```python
from build123d import *

# Parameters (mm, degrees)
SKETCH_1_R           = 4.1
EXTRUDE_1_DEPTH      = 18
EXTRUDE_1_DEPTH_BACK = 18
SKETCH_3_W           = 40
SKETCH_3_H           = 60
EXTRUDE_2_DEPTH      = 4
CUT_EXTRUDE_START    = 50
SKETCH_4_W           = 18
SKETCH_4_H           = 20
CUT_EXTRUDE_1_DEPTH  = 29
SKETCH_5_R           = 6
CUT_EXTRUDE_2_DEPTH  = 55
EXTRUDE_START        = 18
EXTRUDE_3_DEPTH      = 4
EXTRUDE_START_2      = -18
EXTRUDE_4_DEPTH      = 4
SKETCH_7_R           = 2.5
CUT_EXTRUDE_4_DEPTH  = 5
FILLET_1_R           = 2


with BuildPart() as part:
    # Эскиз1 → Бобышка-Вытянуть1 (new body, two sides)
    with BuildSketch(Plane.XY) as extrude_1_sk:
        with BuildLine():
            Line((-9, 0), (-9, -73))
            Line((-9, -73), (9, -73))
            Line((9, -73), (9, 0))
            ThreePointArc((9, 0), (0, 9), (-9, 0))
        make_face()
        Circle(SKETCH_1_R, mode=Mode.SUBTRACT)
    extrude(amount=EXTRUDE_1_DEPTH)
    extrude(extrude_1_sk.sketch, amount=-EXTRUDE_1_DEPTH_BACK)

    # Эскиз3 → Бобышка-Вытянуть2 (add)
    with BuildSketch(Plane.XZ.offset(73)):
        Rectangle(SKETCH_3_W, SKETCH_3_H)
    extrude(amount=-EXTRUDE_2_DEPTH)

    # Эскиз4 → Вырез-Вытянуть1 (cut, through all)
    with BuildSketch(Plane(origin=(0, -69, 0), x_dir=(1, 0, 0), z_dir=(0, 1, 0)).offset(CUT_EXTRUDE_START)):
        Rectangle(SKETCH_4_W, SKETCH_4_H)
    extrude(amount=CUT_EXTRUDE_1_DEPTH, mode=Mode.SUBTRACT)

    # Эскиз5 → Вырез-Вытянуть2 (cut, through all)
    with BuildSketch(Plane(origin=(0, -19, 0), x_dir=(1, 0, 0), z_dir=(0, 1, 0))):
        Circle(SKETCH_5_R)
    extrude(amount=-CUT_EXTRUDE_2_DEPTH, mode=Mode.SUBTRACT)

    # Эскиз6 → Бобышка-Вытянуть3 (add)
    with BuildSketch(Plane.XY.offset(EXTRUDE_START)):
        Polygon((-20, -69), (-9, -34.5), (-9, -69), align=None)
        Polygon((9, -34.5), (20, -69), (9, -69), align=None)
    extrude(amount=-EXTRUDE_3_DEPTH)

    # Эскиз6<3> → Бобышка-Вытянуть4 (add)
    with BuildSketch(Plane.XY.offset(EXTRUDE_START_2)):
        Polygon((-20, -69), (-9, -34.5), (-9, -69), align=None)
        Polygon((9, -34.5), (20, -69), (9, -69), align=None)
    extrude(amount=EXTRUDE_4_DEPTH)

    # Эскиз7 → Вырез-Вытянуть4 (cut, through all)
    with BuildSketch(Plane(origin=(0, -69, 0), x_dir=(1, 0, 0), z_dir=(0, 1, 0))):
        with Locations((-14, -24)):
            Circle(SKETCH_7_R)
        with Locations((-14, 24)):
            Circle(SKETCH_7_R)
        with Locations((14, 24)):
            Circle(SKETCH_7_R)
        with Locations((14, -24)):
            Circle(SKETCH_7_R)
    extrude(amount=-CUT_EXTRUDE_4_DEPTH, mode=Mode.SUBTRACT)

    # Скругление1
    fillet_1_edges = [part.edges().sort_by_distance(p)[0] for p in [
        (-20, -71, -30),
        (0, -69, 30),
        (-20, -71, 30),
        (20, -71, 30),
        (0, -69, -30),
        (20, -71, -30),
        (0, -19, -10),
        (0, -19, 10),
    ]]
    fillet(fillet_1_edges, radius=FILLET_1_R)


solid = part.part
```
Check sheet for the modelled part. Datum: model origin and axes. Units: mm. A direction names the side the tool comes from. Round coordinates to 2 decimals unless told otherwise and drop trailing zeros. Order: outer loops, then holes, each group sorted by start corner. A loop starts at its lowest first (then second) coordinate and runs counter-clockwise, first axis right, second up. Notation, with made-up numbers: (45, 30.25) -> (63, 30.25) arc R12 cw to (63, 46.25) -> close; hole circle Ø5 at (2, 26). An arc over 180 degrees is marked (long way). Use CSV: the item, a comma, the result in double quotes.
(1) Cross-section at D-D (x = -0.5). Record the boundary of the cut face in (y, z).
Worked out:
outline,"(-73, -30) -> (-71, -30) arc R2 ccw to (-69, -28) -> (-69, -18) -> (-4.07, -18) -> (-4.07, -10) -> (-17, -10) arc R2 cw to (-19, -8) -> (-19, -5.98) -> (-73, -5.98) -> close; (-73, 5.98) -> (-19, 5.98) -> (-19, 8) arc R2 cw to (-17, 10) -> (-4.07, 10) -> (-4.07, 18) -> (-69, 18) -> (-69, 28) arc R2 ccw to (-71, 30) -> (-73, 30) -> close; (4.07, -18) -> (8.99, -18) -> (8.99, -10) -> (4.07, -10) -> close; (4.07, 10) -> (8.99, 10) -> (8.99, 18) -> (4.07, 18) -> close"
(2) Draft check along Y on faces 5 (the face through (0, -73, 7)), 6 (the face through (0, -72, 30)), 7 (the face through (-14.577, -51.992, -16.028)), 8 (the face through (-0.534, 4.065, 13.944)). Enter one of: pulls with the +Y half, pulls with the -Y half, needs draft (parallel to the pull), parting line crosses it, or undercut.
Worked out:
face 5,"pulls with the -Y half"
face 6,"needs draft"
face 7,"pulls with the +Y half"
face 8,"undercut"
(3) Cross-section at A-A (z = 24). Record the boundary of the cut face in (x, y).
Worked out:
outline,"(-20, -73) -> (-16.5, -73) -> (-16.5, -69) -> (-20, -69) -> close; (-11.5, -73) -> (11.5, -73) -> (11.5, -69) -> (-11.5, -69) -> close; (16.5, -73) -> (20, -73) -> (20, -69) -> (16.5, -69) -> close"
(4) Material ranges on line 1 along X through (y, z) = (-70, 24); line 2 along Z through (x, y) = (0, -58); line 3 along Y through (x, z) = (0, 15.75), recorded low to high. Write a range as from..to.
Worked out:
line 1,"-20..-16.5, -11.5..11.5, 16.5..20"
line 2,"-18..-6, 6..18"
line 3,"-73..-4.1, 4.1..9"
(5) Cross-section at B-B (y = -15). Record the boundary of the cut face in (x, z).
Worked out:
outline,"(-9, -18) -> (9, -18) -> (9, -10) -> (-9, -10) -> close; (-9, 10) -> (9, 10) -> (9, 18) -> (-9, 18) -> close"
(6) Cross-section at C-C (z = 0). Record the boundary of the cut face in (x, y).
Worked out:
outline,"(-20, -73) -> (-6, -73) -> (-6, -19) -> (-9, -19) -> (-9, -69) -> (-20, -69) -> close; (6, -73) -> (20, -73) -> (20, -69) -> (9, -69) -> (9, -19) -> (6, -19) -> close"
(7) Depth check by flat-ended pin: pin 1 (9 mm diameter, centred on x = -12.5, y = -59.5, fed in from +Z); pin 2 (3 mm diameter, centred on x = 14, z = -24, fed in from +Y); pin 3 (8 mm diameter, centred on x = 9.5, z = -19, fed in from +Y); pin 4 (12 mm diameter, centred on x = 14.5, z = 2.5, fed in from +Y). Enter the tip coordinate at first touch or a pass-through.
Worked out:
pin 1,"z = 18"
pin 2,"through"
pin 3,"y = 7.02"
pin 4,"y = -19"
(8) Tool access check on faces 1 (the face through (12, -59, -14)), 2 (the face through (0, -69, -23)), 3 (the face through (-12, -59, -14)), 4 (the face through (0.13, -18.4, -9.43)). Record the directions out of +Z, -Z, +X, -X, +Y, -Y that give a thin tool (end or side, any length) a straight path to the whole face; none if there is none.
Worked out:
face 1,"+X, +Y"
face 2,"-Z, +X, -X, +Y"
face 3,"-X, +Y"
face 4,"+X, -X, +Y"
